from build123d import *

# Parameters (mm, degrees)
F1_DEPTH = 1
F2_R     = 1.375
F3_DEPTH = 2
F4_R     = 0.5


with BuildPart() as f1:
    # F0 (on Top) → F1 (new body, symmetric)
    with BuildSketch(Plane.XY):
        Polygon((-20.375, 25.5), (-20.375, 0), (20.375, 0), (20.375, 25.5), (16, 36.5), (-16, 36.5), align=None)
    extrude(amount=F1_DEPTH, both=True)

    # F2 (on face) → F3 (join)
    with BuildSketch(Plane.XY.offset(1)):
        with Locations((17.625, 6.5)):
            Circle(F2_R)
        with Locations((-17.625, 23)):
            Circle(F2_R)
    extrude(amount=F3_DEPTH)

    # F4
    f4_edges = [f1.edges().sort_by_distance(p)[0] for p in [
        (20.375, 0, 0),
        (-20.375, 0, 0),
        (-16, 36.5, 0),
        (16, 36.5, 0),
    ]]
    fillet(f4_edges, radius=F4_R)


solid = f1.part
Verification items for the finished model (mm, model axes). A direction names the side the tool comes from. Give positions to 0.01 mm unless a question says otherwise; leave off trailing zeros. Write each loop counter-clockwise with the first axis right and the second up, starting at its lowest first coordinate (ties: lowest second). Pieces come first, ordered by that corner, then holes. Notation, with made-up numbers: (16, 46.25) - (54, 46.25) arc R21 cw to (54, 58.25) - close; hole circle Ø4 at (89, 5.5). An arc over 180 degrees is marked (long way). Answer as CSV lines item,"result". Start each with the question number.
1. Sectioned sample at A-A (z = 2). Record the boundary of the cut face in (x, y) (3 decimals), then the cut area to 3 significant figures.
2. Draft check along Z on faces 1 (the face through (-18, 23, 3)), 2 (the face through (0, 0, 0)), 3 (the face through (0, 19, -1)). Enter one of: pulls with the +Z half, pulls with the -Z half, needs draft (parallel to the pull), parting line crosses it, or undercut.
3. Set-up check for faces 4 (the face through (-18.64, 23.93, 1.99)), 5 (the face through (20.375, 13, 0)): record each of +Z, -Z, +X, -X, +Y, -Y from which the full face is reachable in a straight line by a thin tool's end or side.
4. Thickness scan on line 1 (Z direction, x = -14.5, y = 34); line 2 (X direction, y = 7, z = 2.2); line 3 (X direction, y = 28, z = -0.25). Record the ranges inside material, lowest first.
5. Sectioned sample at B-B (y = 23). Record the boundary of the cut face in (x, z) (3 decimals), then the cut area to 3 significant figures.
6. Sectioned sample at C-C (x = 3). Record the boundary of the cut face in (y, z).
7. Sectioned sample at D-D (y = 10). Record the boundary of the cut face in (x, z) (3 decimals), then the cut area to 3 significant figures.
Derived:
1,outline,"circle Ø2.75 at (-17.625, 23); circle Ø2.75 at (17.625, 6.5)"
1,area,"11.9 mm²"
2,face 1,"pulls with the +Z half"
2,face 2,"needs draft"
2,face 3,"pulls with the -Z half"
3,face 4,"+Z"
3,face 5,"+Z, -Z, +X, +Y, -Y"
4,line 1,"-1 to 1"
4,line 2,"16.34 to 18.91"
4,line 3,"-19.38 to 19.38"
5,outline,"(-20.375, -1) - (20.375, -1) - (20.375, 1) - (-16.25, 1) - (-16.25, 3) - (-19, 3) - (-19, 1) - (-20.375, 1) - close"
5,area,"87.0 mm²"
6,outline,"(0, -1) - (36.5, -1) - (36.5, 1) - (0, 1) - close"
7,outline,"(-20.375, -1) - (20.375, -1) - (20.375, 1) - (-20.375, 1) - close"
7,area,"81.5 mm²"
